from build123d import *

# Parameters (mm, degrees)
F0_R     = 60
F1_DEPTH = 3
F2_R     = 40
F3_DEPTH = 57
F4_R     = 60
F4_R_2   = 40
F5_DEPTH = 3
F6_R     = 26.5
F7_DEPTH = 63
F8_R     = 1.5
F9_DEPTH = 25


with BuildPart() as f1:
    # F0 (on Top) → F1 (new body)
    with BuildSketch(Plane.XY):
        Circle(F0_R)
    extrude(amount=F1_DEPTH)

    # F2 (on face) → F3 (join)
    with BuildSketch(Plane.XY.offset(3)):
        Circle(F2_R)
    extrude(amount=F3_DEPTH)

    # F4 (on face) → F5 (join)
    with BuildSketch(Plane.XY.offset(60)):
        Circle(F4_R)
        Circle(F4_R_2, mode=Mode.SUBTRACT)
        Circle(F4_R_2)
    extrude(amount=F5_DEPTH)

    # F6 (on face) → F7 (cut)
    with BuildSketch(Plane.XY.offset(63)):
        Circle(F6_R)
    extrude(amount=-F7_DEPTH, mode=Mode.SUBTRACT)

    # F8 (on face) → F9 (cut)
    with BuildSketch(Plane.XY.offset(63)):
        with Locations((-49.5205215438, -6.9078177476)):
            Circle(F8_R)
        with Locations((-49.9578443444, 2.0527514366)):
            Circle(F8_R)
        with Locations((-48.7868632446, 10.9472359411)):
            Circle(F8_R)
        with Locations((-47.4889736721, -15.6460020316)):
            Circle(F8_R)
        with Locations((-43.928602798, -23.8804911217)):
            Circle(F8_R)
        with Locations((-38.9540287263, -31.3461902947)):
            Circle(F8_R)
        with Locations((-32.7253990171, -37.8027546506)):
            Circle(F8_R)
        with Locations((-25.4432333202, -43.0423265892)):
            Circle(F8_R)
        with Locations((-17.341968002, -46.8962274156)):
            Circle(F8_R)
        with Locations((-8.6824088833, -49.2403876506)):
            Circle(F8_R)
        with Locations((0, -50)):
            Circle(F8_R)
        with Locations((8.9350601107, -49.1951694866)):
            Circle(F8_R)
        with Locations((17.5824718607, -46.8065880328)):
            Circle(F8_R)
        with Locations((25.6638472166, -42.9111517679)):
            Circle(F8_R)
        with Locations((32.9190206792, -37.6342673307)):
            Circle(F8_R)
        with Locations((44.0506097143, -23.6546778418)):
            Circle(F8_R)
        with Locations((47.568663586, -15.4020207974)):
            Circle(F8_R)
        with Locations((49.5553289803, -6.6535231008)):
            Circle(F8_R)
        with Locations((39.1144248494, -31.1458146258)):
            Circle(F8_R)
        with Locations((49.9466487401, 2.3091729323)):
            Circle(F8_R)
        with Locations((48.7300250221, 11.1975292519)):
            Circle(F8_R)
        with Locations((45.9446248618, 19.7254010429)):
            Circle(F8_R)
        with Locations((41.6801192611, 27.618248648)):
            Circle(F8_R)
        with Locations((36.073796389, 34.6219758836)):
            Circle(F8_R)
        with Locations((21.5950281924, 45.0960614396)):
            Circle(F8_R)
        with Locations((29.3061418343, 40.5111102142)):
            Circle(F8_R)
        with Locations((13.1887010456, 48.2292252139)):
            Circle(F8_R)
        with Locations((-13.4361023015, 48.1608882284)):
            Circle(F8_R)
        with Locations((-4.6134179732, 49.7867088148)):
            Circle(F8_R)
        with Locations((4.3577871374, 49.8097349046)):
            Circle(F8_R)
        with Locations((-29.513711345, 40.3601392793)):
            Circle(F8_R)
        with Locations((-21.8262352253, 44.9846135461)):
            Circle(F8_R)
        with Locations((-36.2510460467, 34.4363421478)):
            Circle(F8_R)
        with Locations((-41.8213428283, 27.4039282592)):
            Circle(F8_R)
        with Locations((-46.0452758972, 19.4892936646)):
            Circle(F8_R)
    extrude(amount=-F9_DEPTH, mode=Mode.SUBTRACT)


solid = f1.part
The model under review builds one solid part; all positions refer to its coordinate system, in mm. Coordinates: 2 decimals unless noted, no trailing zeros. Write each loop counter-clockwise with the first axis right and the second up, starting at its lowest first coordinate (ties: lowest second). Pieces come first, ordered by that corner, then holes. Notation, with made-up numbers: (-12, 15) -> (19, 15) arc R31 cw to (19, 39) -> close; hole circle Ø9 at (67.25, 64.5). An arc over 180 degrees is marked (long way). Answer in a Markdown table with one row per item.
1. Clearance check with flat-ended pins moving along their axes: pin 1 Ø2.5 at (x, y) = (29.31, 40.51) entering from +Z; pin 2 Ø10 at (x, z) = (38, 41) entering from +Y; pin 3 Ø1 at (y, z) = (-31, 50.5) entering from -X; pin 4 Ø6 at (x, z) = (-43.5, 37) entering from -Y. State where each tip first meets the part, or that it passes through.
Answers below:
| item | result |
|---|---|
| pin 1 | stops at z = 3 |
| pin 2 | stops at y = 22.61 |
| pin 3 | stops at x = -25.88 |
| pin 4 | passes through |
2. Wall thickness on probe 1 along Z at (x, y) = (-50.5, 13); probe 2 along Y at (x, z) = (-2.5, 9.5); probe 3 along X at (y, z) = (-10.5, 40.5): over which ranges is each line inside the solid? List them lowest first. Write a range as [from, to].
Answers below:
| item | result |
|---|---|
| probe 1 | z = [0, 3], [60, 63] |
| probe 2 | y = [-39.92, -26.38], [26.38, 39.92] |
| probe 3 | x = [-38.6, -24.33], [24.33, 38.6] |
3. We need section B-B, the plane z = 5. State the section outline as (x, y) points.
Answers below:
| item | result |
|---|---|
| outline | circle Ø80 at (0, 0); hole circle Ø53 at (0, 0) |
4. We need section A-A, the plane x = 0. State the section outline as (y, z) points, and give its area (3 significant figures).
Answers below:
| item | result |
|---|---|
| outline | (-60, 0) -> (-26.5, 0) -> (-26.5, 63) -> (-48.5, 63) -> (-48.5, 60) -> (-40, 60) -> (-40, 3) -> (-60, 3) -> close; (-60, 60) -> (-51.5, 60) -> (-51.5, 63) -> (-60, 63) -> close; (26.5, 0) -> (60, 0) -> (60, 3) -> (40, 3) -> (40, 60) -> (60, 60) -> (60, 63) -> (26.5, 63) -> close |
| area | 1,930 mm^2 |
5. Draft analysis for pull direction X (two halves, no side actions). For faces 1 (the flat face through (26, -12, 63)), 2 (the cylindrical face through (24.558, -41.897, 61.521)), state which applies: +X half, -X half, draft (parallel to the pull), parting line (faces both ways), or undercut.
Answers below:
| item | result |
|---|---|
| face 1 | draft |
| face 2 | undercut |
